Input: part model. Units: mm. Frame: model coordinates. A direction names the side the tool comes from. Give positions to 0.01 mm unless a question says otherwise; leave off trailing zeros. Write each loop counter-clockwise with the first axis right and the second up, starting at its lowest first coordinate (ties: lowest second). Pieces come first, ordered by that corner, then holes. Notation, with made-up numbers: (-26.75, -13.75) - (-17.75, -13.75) arc R20 cw to (-17.75, 0.25) - close; hole circle Ø7 at (-1, -7). An arc over 180 degrees is marked (long way). Use a Markdown table: item, result. Add a question column.
1. Material intervals for probe 1 along Y at (x, z) = (0, 7.5); probe 2 along X at (y, z) = (-1, 1.5); probe 3 along X at (y, z) = (-0.75, 5), sorted ascending.
2. Set-up query: faces 3 (the cylindrical face through (21.491, -2.085, 5.067)), 4 (the flat face through (12, 0, 0)), 5 (the cylindrical face through (2.976, 2.096, 5.067)). Return all of +Z, -Z, +X, -X, +Y, -Y with unobstructed straight access to the full face (end or side cutting, diameter ignored); none if empty.
3. Mould query, pull axis X, two halves, no side actions, for faces 1 (the flat face through (12, 1.9, 5)), 2 (the flat face through (12, 0, 10)). Classes: released by +X, released by -X, zero draft, split by the parting line, or undercut.
4. Section query B-B, the plane y = 0. Return loops of the section in (x, z), plus the area to 3 significant figures.
5. Pin query (flat end, axial travel): pin 1 (4 mm diameter, centred on x = 22, z = 4.5, fed in from +Y); pin 2 (3 mm diameter, centred on x = 0, y = 0, fed in from +Z); pin 3 (5 mm diameter, centred on x = 14, z = 6.5, fed in from -Y); pin 4 (1.5 mm diameter, centred on x = 11.5, z = 2, fed in from +Y). Return the tip coordinate at first contact, or that it passes through.
6. Section query C-C, the plane z = 8.75. Return loops of the section in (x, y), plus the area to 3 significant figures.
7. Section query A-A, the plane x = 0. Return loops of the section in (y, z).
```python
from build123d import *

# Parameters (mm, degrees)
F1_DEPTH = 10
F2_D     = 2.6
F3_R     = 4
F4_SIZE  = 0.2


with BuildPart() as f1:
    # F0 (on Top) → F1 (new body)
    with BuildSketch(Plane.XY):
        with BuildLine():
            ThreePointArc((2.636759, 1.9), (-3.25, 0), (2.636759, -1.9))
            Line((2.636759, -1.9), (21.863241, -1.9))
            ThreePointArc((21.863241, -1.9), (27.75, 0), (21.863241, 1.9))
            Line((21.863241, 1.9), (2.636759, 1.9))
        make_face()
    extrude(amount=F1_DEPTH)

    # F2 (through all)
    with Locations(Plane(origin=(0, 0, 0), x_dir=(1, 0, 0), z_dir=(0, 0, -1))):
        with Locations((0, 0), (24.5, 0)):
            Hole(F2_D / 2)

    # F3
    f3_edges = [f1.edges().sort_by_distance(p)[0] for p in [
        (2.636759, -1.9, 5),
        (21.863241, -1.9, 5),
        (2.636759, 1.9, 5),
        (21.863241, 1.9, 5),
    ]]
    fillet(f3_edges, radius=F3_R)

    # F4
    f4_edges = [f1.edges().sort_by_distance(p)[0] for p in [
        (12.25, 1.9, 0),
        (12.25, 1.9, 10),
    ]]
    chamfer(f4_edges, length=F4_SIZE)


solid = f1.part
```
Result sheet:
| question | item | result |
|---|---|---|
| 1 | probe 1 | y = -3.25 to -1.3, 1.3 to 3.25 |
| 1 | probe 2 | x = -3.09 to -0.83, 0.83 to 23.67, 25.33 to 27.59 |
| 1 | probe 3 | x = -3.16 to -1.06, 1.06 to 23.44, 25.56 to 27.66 |
| 2 | face 3 | +Z, -Z, -Y |
| 2 | face 4 | -Z, +X, -X, +Y, -Y |
| 2 | face 5 | +Z, -Z, +Y |
| 3 | face 1 | undercut |
| 3 | face 2 | zero draft |
| 4 | outline | (-3.25, 0.2) - (-3.05, 0) - (-1.3, 0) - (-1.3, 10) - (-3.05, 10) - (-3.25, 9.8) - close; (1.3, 0) - (23.2, 0) - (23.2, 10) - (1.3, 10) - close; (25.8, 0) - (27.55, 0) - (27.75, 0.2) - (27.75, 9.8) - (27.55, 10) - (25.8, 10) - close |
| 4 | area | 258 mm² |
| 5 | pin 1 | stops at y = 3.21 |
| 5 | pin 2 | stops at z = 10 |
| 5 | pin 3 | stops at y = -1.9 |
| 5 | pin 4 | stops at y = 1.9 |
| 6 | outline | (1.89, -2.64) arc R4 cw to (4.21, -1.9) - (20.29, -1.9) arc R4 cw to (22.61, -2.64) arc R3.25 ccw (long way) to (22.61, 2.64) arc R4 cw to (20.29, 1.9) - (4.21, 1.9) arc R4 cw to (1.89, 2.64) arc R3.25 ccw (long way) to start; hole circle Ø2.6 at (0, 0); hole circle Ø2.6 at (24.5, 0) |
| 6 | area | 127 mm² |
| 7 | outline | (-3.25, 0.2) - (-3.05, 0) - (-1.3, 0) - (-1.3, 10) - (-3.05, 10) - (-3.25, 9.8) - close; (1.3, 0) - (3.05, 0) - (3.25, 0.2) - (3.25, 9.8) - (3.05, 10) - (1.3, 10) - close |
